For this review, take the finished solid that the model builds, in its own axes (mm). Round coordinates to 2 decimals unless told otherwise and drop trailing zeros. Loops run counter-clockwise (first coordinate to the right, second up) from the corner with the lowest first, then second, coordinate; pieces in that order, holes last. Notation, with made-up numbers: (-14.5, 89.25) -> (9.5, 89.25) arc R19 cw to (9.5, 98.25) -> close; hole circle Ø3 at (53, 22). An arc over 180 degrees is marked (long way). One line per question, with ' | ' between items. Start each with the question number.
1. Consider section A-A (x = -5.5). Write out the cut boundary in (y, z), and give its area (3 significant figures).
2. For pin 1 Ø3 at (x, y) = (-6, 5) entering from -Z; pin 2 Ø1 at (y, z) = (5.5, -2) entering from +X, all flat-tipped, find the tip position at first contact; note any pin that passes through.
3. Consider section C-C (y = 7.75). Write out the cut boundary in (x, z).
4. Wall thickness on line 1 along Z through (x, y) = (-6.25, 9); line 2 along Z through (x, y) = (-6, 4.5); line 3 along X through (y, z) = (6.5, -6.5): over which ranges is each line inside the solid? List them lowest first.
5. Consider section B-B (z = -6.25). Write out the cut boundary in (x, y).
6. Draft analysis for pull direction Z (two halves, no side actions). For faces 1 (the face through (-4.93, 5.771, -8.782)), 2 (the face through (-5, 1, 0)), 3 (the face through (0, 1, -5)), 4 (the face through (-6.1, 5.07, -4.26)), state which applies: pulls with the +Z half, pulls with the -Z half, needs draft (parallel to the pull), parting line crosses it, or undercut.
7. Consider section D-D (x = -8.75). Write out the cut boundary in (y, z).
Autodesk Inventor part; units mm, degrees
ref_plane "YZ Plane" through (0, 0, 0) normal (1, 0, 0) x (0, 1, 0)
ref_plane "XZ Plane" through (0, 0, 0) normal (0, 1, 0) x (-1, 0, 0)
ref_plane "XY Plane" through (0, 0, 0) normal (0, 0, 1) x (1, 0, 0)
sketch "Sketch3" plane through (0, 0, 0) normal (0, 1, 0) x (-1, 0, 0)
  line L0 (10, 0) -> (10, -10)
  line L1 (10, -10) -> (0, -10)
  line L2 (0, -10) -> (0, 0)
  line L3 (0, 0) -> (10, 0)
  dimension "d0" = 10
  dimension "d1" = 10
extrude "Extrusion1" add sketch "Sketch3" along normal blind 10
sketch "Sketch4" plane through (0, 0, 0) normal (1, 0, 0) x (0, 0, -1)
  line L0 (10, 10) -> (0, 10)
  line L1 (3.4236, 10) -> (0, 3)
  line L2 (0, 0) -> (0, 10)
  line L3 (6.9236, 10) -> (10, 3)
  line L4 (10, 0) -> (10, 10)
  line L5 (3.4236, 10) -> (6.9236, 10)
  dimension "d4" = 3.5
  dimension "d5" = 7
  dimension "d6" = 7
extrude "Extrusion2" cut sketch "Sketch4" against normal blind 10
sketch "Sketch6" plane through (-10, 0, 0) normal (0, 0, 1) x (1, 0, 0)
  line L0 (0, 10) -> (10, 10)
  line L1 (3.3385, 10) -> (0, 3)
  line L2 (0, 3) -> (0, 10)
  line L3 (3.3385, 10) -> (6.8385, 10)
  line L4 (6.8385, 10) -> (10, 3)
  line L5 (10, 10) -> (10, 3)
  point P0 (10, 0)
  dimension "d12" = 3.5
  dimension "d13" = 7
  dimension "d14" = 7
extrude "Extrusion3" cut sketch "Sketch6" against normal blind 10
sketch "Sketch7" plane through (0, 10, 0) normal (0, 1, 0) x (1, 0, 0)
  circle A0 centre (-4.9115, 5.1736) radius 1.5
  line L0 (-6.6615, 3.4236) -> (-3.1615, 3.4236)
  point P0 (0, 0)
  dimension "d17" = 1.75
  dimension "d18" = 3
extrude "Extrusion4" cut sketch "Sketch7" against normal blind 10
properties part number "Stand"
Answer block:
1) outline: (0, -10) -> (3, -10) -> (10, -6.92) -> (10, -6.55) -> (0, -6.55) -> close; (0, -3.79) -> (10, -3.79) -> (10, -3.42) -> (3, 0) -> (0, 0) -> close | area: 49.7 mm2
2) pin 1: stops at z = -9.78 | pin 2: stops at x = -0.9
3) outline: (-7.73, -7.91) -> (-2.15, -7.91) -> (-2.15, -2.32) -> (-7.73, -2.32) -> close; hole circle Ø3 at (-4.91, -5.17)
4) line 1: z = -7.36 to -5.85, -4.5 to -2.93 | line 2: z = -9.34 to -6.21, -4.14 to -0.73 | line 3: x = -8.33 to -5.61, -4.21 to -1.58
5) outline: (-10, 0) -> (-5.96, 0) -> (-5.96, 10) -> (-6.66, 10) -> (-10, 3) -> close; (-3.87, 0) -> (0, 0) -> (0, 3) -> (-3.16, 10) -> (-3.87, 10) -> close
6) face 1: pulls with the -Z half | face 2: pulls with the +Z half | face 3: needs draft | face 4: undercut
7) outline: (0, -10) -> (3, -10) -> (5.62, -8.85) -> (5.62, -1.28) -> (3, 0) -> (0, 0) -> close
